Autodesk Inventor part; units mm, degrees
ref_plane "IP1_XY" through (0, 0, 0) normal (1, 0, 0) x (0, 0, -1)
ref_plane "IP1_YZ" through (0, 0, 0) normal (0, 0, -1) x (0, 1, 0)
ref_plane "IP1_ZX" through (0, 0, 0) normal (0, 1, 0) x (1, 0, 0)
sketch "Skizze_2" plane through (0, 0, 0) normal (0, 0, 1) x (1, 0, 0)
  line L0 (8, 0) -> (-6, 0)
  line L1 (-0.4283, 0) -> (-1.15, 1.25)
  line L2 (-1.15, 1.25) -> (-2.815, 1.25)
  line L3 (-2.815, 1.25) -> (-3, 1.435)
  line L4 (-3, 1.435) -> (-3, 2.45)
  arc A0 (-2.7, 2.75) -> (-3, 2.45) centre (-2.7, 2.45) ccw
  line L5 (-2.7, 2.75) -> (0, 2.75)
  line L6 (0, 2.75) -> (0, 1.8)
  arc A1 (0, 1.8) -> (0.0562, 1.7101) centre (0.1, 1.8) ccw
  line L7 (0.0562, 1.7101) -> (0.4662, 1.5101)
  arc A2 (0.4662, 1.5101) -> (0.51, 1.5) centre (0.51, 1.6) ccw
  line L8 (0.51, 1.5) -> (7.6935, 1.5)
  line L9 (7.6935, 1.5) -> (8, 1.1935)
  line L10 (8, 1.1935) -> (8, 0)
  line L11 (8, 0) -> (-0.4283, 0)
revolve "Revolution1" add sketch "Skizze_2" angle 360 about axis through (8, 0, 0) along (1, 0, 0)
thread "Thread1"
sketch "Skizze_1" plane through (-1.15, 0, 0) normal (1, 0, 0) x (0, 0, -1)
  line L0 (-1.25, -0.7217) -> (0, -1.4434)
  line L1 (0, -1.4434) -> (1.25, -0.7217)
  line L2 (1.25, -0.7217) -> (1.25, 0.7217)
  line L3 (1.25, 0.7217) -> (0, 1.4434)
  line L4 (0, 1.4434) -> (-1.25, 0.7217)
  line L5 (-1.25, 0.7217) -> (-1.25, -0.7217)
extrude "Extrusion1" cut sketch "Skizze_1" against normal blind 2.6
ref_plane "IP1_XY" through (0, 0, 0) normal (1, 0, 0) x (0, 0, -1)
ref_plane "IP1_YZ" through (0, 0, 0) normal (0, 0, -1) x (0, 1, 0)
ref_plane "IP1_ZX" through (0, 0, 0) normal (0, 1, 0) x (1, 0, 0)
ref_plane "IP2_XY" through (-3, 0, 0) normal (1, 0, 0) x (0, 0, -1)
ref_plane "IP2_YZ" through (-3, 0, 0) normal (0, 0, -1) x (0, 1, 0)
ref_plane "IP2_ZX" through (-3, 0, 0) normal (0, 1, 0) x (1, 0, 0)
ref_plane "IP3_XY" through (8, 0, 0) normal (1, 0, 0) x (0, 0, -1)
ref_plane "IP3_YZ" through (8, 0, 0) normal (0, 0, -1) x (0, 1, 0)
ref_plane "IP3_ZX" through (8, 0, 0) normal (0, 1, 0) x (1, 0, 0)
properties part number "M3x8_p3"
Could you check a few things on this model? Use its own coordinates, in mm. A direction names the side the tool comes from. Give positions to 0.01 mm unless a question says otherwise; leave off trailing zeros. Write each loop counter-clockwise with the first axis right and the second up, starting at its lowest first coordinate (ties: lowest second). Pieces come first, ordered by that corner, then holes. Notation, with made-up numbers: (20, 74) -> (46, 74) arc R12 ccw to (46, 82) -> close; hole circle Ø2 at (12, 67). An arc over 180 degrees is marked (long way). Answer as a JSON object with one key per item and string values.
Q1. Please list where these lines run through material, in increasing order: L1, parallel to Z at x = -2, y = 0.1; L2, parallel to X at y = -1.25, z = 1.45; L3, parallel to Y at x = -2.5, z = 0.85.
Taken from the geometry:
{"L1": "z = -2.75 to -1.25, 1.25 to 2.75", "L2": "x = -3 to 0", "L3": "y = -2.62 to -0.95, 0.95 to 2.62"}
Q2. Will these pins go through, and if not, where does the flat tip stop? pin 1 Ø2 at (x, y) = (5.5, -1.5) entering from +Z; pin 2 Ø0.7 at (x, y) = (-2, -0.5) entering from +Z.
Taken from the geometry:
{"pin 1": "stops at z = 1.41", "pin 2": "stops at z = 2.75"}
Q3. Which directions (+Z, -Z, +X, -X, +Y, -Y) give clear straight access to the entire face, cutting with the end or side of a thin tool? Please do faces 1 (the flat face through (-2.062, 1.088, 0.616)), 2 (the flat face through (0, 2, -1)), 3 (the cylindrical face through (-1.331, -0.596, -2.685)).
Taken from the geometry:
{"face 1": "-X", "face 2": "+X", "face 3": "+X, -X"}
Q4. Suppose I cut it at A-A on x = -0.25. Write out the boundary of the cut face in (y, z), then the cut area to 3 significant figures.
Taken from the geometry:
{"outline": "circle Ø5.5 at (0, 0)", "area": "23.8 mm²"}
Q5. We'd pull the mould along Y, two halves only. Please class faces 4 (the flat face through (-3, 0, -2)), 5 (the cylindrical face through (4.15, -1.5, 0.07)), 6 (the flat face through (-2.06, 1.08, -0.63)), 7 (the conical face through (-0.55, -0.17, 0.13)): released by +Y, released by -Y, zero draft, split by the parting line, or undercut.
Taken from the geometry:
{"face 4": "zero draft", "face 5": "split by the parting line", "face 6": "undercut", "face 7": "undercut"}
Q6. Suppose I cut it at B-B on x = 5.5. Write out the boundary of the cut face in (y, z).
Taken from the geometry:
{"outline": "circle Ø3 at (0, 0)"}
